Geometry: final body of the model. Coordinates: model frame, mm. Face numbers are marked on the shaded views. A direction names the side the tool comes from. Give positions to 0.01 mm unless a question says otherwise; leave off trailing zeros. Loops run counter-clockwise (first coordinate to the right, second up) from the corner with the lowest first, then second, coordinate; pieces in that order, holes last.
Autodesk Inventor part; units mm, degrees
ref_plane "YZ Plane" through (0, 0, 0) normal (1, 0, 0) x (0, 1, 0)
ref_plane "XZ Plane" through (0, 0, 0) normal (0, 1, 0) x (-1, 0, 0)
ref_plane "XY Plane" through (0, 0, 0) normal (0, 0, 1) x (1, 0, 0)
sketch "Sketch1" plane through (0, 0, 0) normal (0, 0, 1) x (1, 0, 0)
  circle A0 centre (0, 0) radius 15
  circle A1 centre (0, 12) radius 1
  circle A2 centre (-8.4853, 8.4853) radius 1
  circle A3 centre (-12, 0) radius 1
  circle A4 centre (-8.4853, -8.4853) radius 1
  circle A5 centre (0, -12) radius 1
  circle A6 centre (8.4853, -8.4853) radius 1
  circle A7 centre (12, 0) radius 1
  circle A8 centre (8.4853, 8.4853) radius 1
  circle A9 centre (0, 0) radius 1.5
  dimension "d0" = 30
  dimension "d1" = 2
  dimension "d4" = 360
  dimension "d6" = 12
  dimension "d9" = 3
extrude "Extrusion1" add sketch "Sketch1" along normal blind 5
sketch "Sketch2" plane through (0, 0, 5) normal (0, 0, 1) x (1, 0, 0)
  point P0 (0, 0)
sketch "Sketch3" plane through (0, 0, 5) normal (0, 0, 1) x (1, 0, 0)
  circle A0 centre (0, 0) radius 6
  circle A1 centre (0, 0) radius 1.5
  dimension "d10" = 12
extrude "Extrusion2" add sketch "Sketch3" along normal blind 1.5
sketch "Sketch4" plane through (0, 0, 0) normal (0, 0, -1) x (-1, 0, 0)
  circle A0 centre (0, 0) radius 1.5
  circle A1 centre (0, 0) radius 3.9
  dimension "d13" = 7.8
extrude "Extrusion3" cut sketch "Sketch4" against normal blind 5.5
properties part number "orczyk serwa okrągły 02-1"
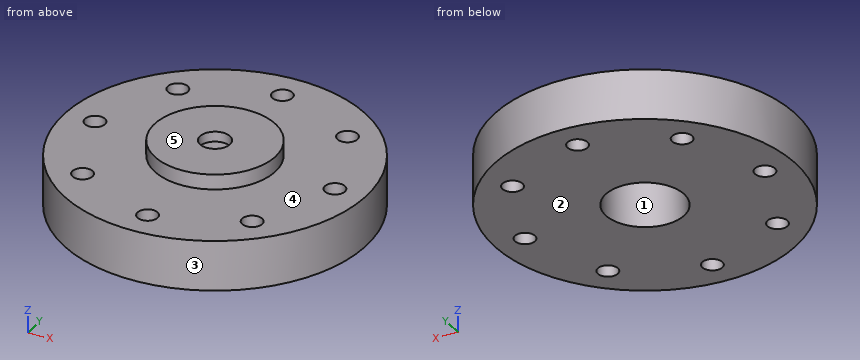
Item 1: Section query A-A on y = 0. Return loops of the section in (x, z).
Values follow:
outline: (-15, 0) - (-13, 0) - (-13, 5) - (-15, 5) - close; (-11, 0) - (-3.9, 0) - (-3.9, 5.5) - (-1.5, 5.5) - (-1.5, 6.5) - (-6, 6.5) - (-6, 5) - (-11, 5) - close; (1.5, 5.5) - (3.9, 5.5) - (3.9, 0) - (11, 0) - (11, 5) - (6, 5) - (6, 6.5) - (1.5, 6.5) - close; (13, 0) - (15, 0) - (15, 5) - (13, 5) - close
Item 2: Set-up query: the marked faces 4 and 5. Return all of +Z, -Z, +X, -X, +Y, -Y with unobstructed straight access to the full face (end or side cutting, diameter ignored); none if empty.
Values follow:
face 4: +Z
face 5: +Z, +X, -X, +Y, -Y
Item 3: Pin query (flat end, axial travel): pin 1 (3 mm diameter, centred on x = 0, y = 12, fed in from +Z); pin 2 (4 mm diameter, centred on x = 0.5, y = -1.5, fed in from -Z). Return the tip coordinate at first contact, or that it passes through.
Values follow:
pin 1: stops at z = 5
pin 2: stops at z = 5.5
Item 4: Section query B-B on x = -12. Return loops of the section in (y, z).
Values follow:
outline: (-9, 0) - (-1, 0) - (-1, 5) - (-9, 5) - close; (1, 0) - (9, 0) - (9, 5) - (1, 5) - close
Item 5: Draft query along Y for the marked faces 1, 2 and 3. Return one class per face: +Y half, -Y half, draft (parallel to the pull), parting line (faces both ways), or undercut.
Values follow:
face 1: undercut
face 2: draft
face 3: parting line
Item 6: Ray query, probe 1 along Y at (x, z) = (0, 1.9); probe 2 along X at (y, z) = (-8.75, 4); probe 3 along Z at (x, y) = (7.75, 5.25). Return the intervals inside material, ascending.
Values follow:
probe 1: y = -15 to -13, -11 to -3.9, 3.9 to 11, 13 to 15
probe 2: x = -12.18 to -9.45, -7.52 to 7.52, 9.45 to 12.18
probe 3: z = 0 to 5
